Build history of the part. All positions in model axes, mm. Face numbers are marked on the shaded views. Round coordinates to 2 decimals unless told otherwise and drop trailing zeros. Loops run counter-clockwise (first coordinate to the right, second up) from the corner with the lowest first, then second, coordinate; pieces in that order, holes last. Notation, with made-up numbers: (8.5, -15) - (12.5, -15) arc R9 ccw to (12.5, -10) - close; hole circle Ø5 at (61.25, 52.25). An arc over 180 degrees is marked (long way). Put each result on its own line as item: value. Start each with the question number.
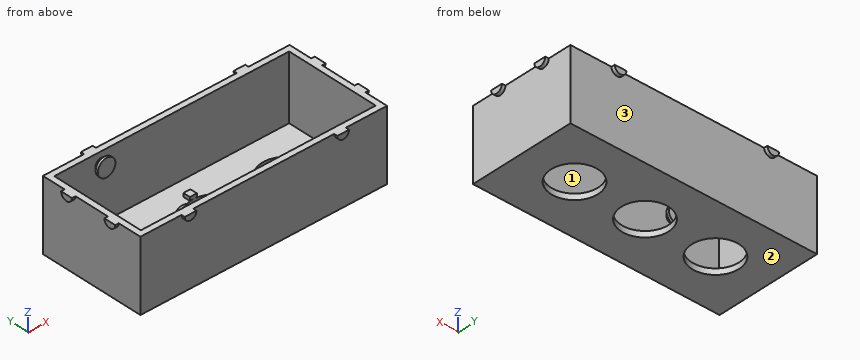
Autodesk Fusion 360 part; units mm, degrees
sketch "Sketch1" plane through (0, 0, 0) normal (0, 0, 1) x (1, 0, 0)
  line L0 (0, 0) -> (210, 0)
  line L1 (210, 0) -> (210, 90)
  line L2 (210, 90) -> (0, 90)
  line L3 (0, 90) -> (0, 0)
  line L4 (5, 5) -> (205, 5)
  line L5 (205, 5) -> (205, 85)
  line L6 (205, 85) -> (5, 85)
  line L7 (5, 85) -> (5, 5)
  circle A0 centre (45, 45) radius 20
  circle A1 centre (105, 45) radius 20
  circle A2 centre (165, 45) radius 20
  dimension "d1" = 210
  dimension "d2" = 90
  dimension "d3" = 200
  dimension "d4" = 80
  dimension "d5" = 5
  dimension "d6" = 5
  dimension "d7" = 40
  dimension "d8" = 40
  dimension "d9" = 40
  dimension "d10" = 105
  dimension "d11" = 45
  dimension "d12" = 45
  dimension "d13" = 45
  dimension "d14" = 60
  dimension "d15" = 60
extrude "Extrude1" add sketch "Sketch1" along normal blind 5 contours L4 L5 L6 L7
extrude "Extrude2" add sketch "Sketch1" along normal blind 60 contours L0 L1 L2 L3
sketch "Sketch2" plane through (210, 0, 0) normal (1, 0, 0) x (0, 1, 0)
  line L0 (0, 0) -> (90, 0)
  line L1 (90, 0) -> (90, 60)
  line L2 (90, 60) -> (0, 60)
  line L3 (0, 60) -> (0, 0)
  circle A0 centre (25, 60) radius 5
  circle A1 centre (65, 60) radius 5
  line L4 (20, 60) -> (30, 60)
  line L5 (60, 60) -> (70, 60)
  dimension "d20" = 10
  dimension "d21" = 10
  dimension "d22" = 25
  dimension "d23" = 25
extrude "Extrude3" add sketch "Sketch2" along normal blind 3 contours L2 A0 L4 | L2 A1 L5 picked at (25.8333, 56.3489) picked at (63.59, 57.0721)
sketch "Sketch3" plane through (0, 0, 0) normal (0, -1, 0) x (1, 0, 0)
  line L0 (0, 0) -> (210, 0)
  line L1 (210, 0) -> (210, 60)
  line L2 (210, 60) -> (0, 60)
  line L3 (0, 60) -> (0, 0)
  circle A0 centre (40, 60) radius 5
  circle A1 centre (170, 60) radius 5
  line L4 (35, 60) -> (45, 60)
  line L5 (165, 60) -> (175, 60)
  dimension "d26" = 10
  dimension "d27" = 10
  dimension "d28" = 40
  dimension "d29" = 40
extrude "Extrude4" add sketch "Sketch3" along normal blind 3 contours L2 A0 L4 | L2 A1 L5 picked at (38.8698, 57.4825) picked at (169.3911, 57.9517)
ref_plane "WorkPlane1" through (105, 45, 30) normal (0, -1, 0) x (1, 0, 0)
ref_plane "WorkPlane2" through (105, 0, 0) normal (1, 0, 0) x (0, 1, 0)
mirror "Mirror1" about plane through (105, 45, 30) normal (0, -1, 0) of bodies 1 merged
mirror "Mirror2" about plane through (105, 0, 0) normal (1, 0, 0) of bodies 1 merged
sketch "Sketch4" plane through (0, 85, 0) normal (0, -1, 0) x (1, 0, 0)
  line L0 (5, 5) -> (205, 5)
  line L1 (205, 5) -> (205, 60)
  line L2 (205, 60) -> (5, 60)
  line L3 (5, 60) -> (5, 5)
  circle A0 centre (45, 50) radius 5
  line L4 (0, 0) -> (0, 60)
  dimension "d38" = 45
  dimension "d39" = 10
extrude "Extrude5" add sketch "Sketch4" along normal blind 5 contours A0
sketch "Sketch5" plane through (0, 80, 0) normal (0, -1, 0) x (1, 0, 0)
  circle A0 centre (45, 50) radius 5
  circle A1 centre (45, 50) radius 7.5
  dimension "d42" = 15
extrude "Extrude6" add sketch "Sketch5" against normal blind 2
mirror "Mirror3" about plane through (105, 45, 30) normal (0, -1, 0) of bodies 1 merged
sketch "Sketch6" plane through (0, 0, 5) normal (0, 0, 1) x (-1, 0, 0)
  arc A0 (-65, -45) -> (-25, -45) centre (-45, -45) ccw
  arc A1 (-25, -45) -> (-65, -45) centre (-45, -45) ccw
  arc A2 (-125, -45) -> (-85, -45) centre (-105, -45) ccw
  arc A3 (-85, -45) -> (-125, -45) centre (-105, -45) ccw
  arc A4 (-185, -45) -> (-145, -45) centre (-165, -45) ccw
  arc A5 (-145, -45) -> (-185, -45) centre (-165, -45) ccw
  line L0 (-5, -85) -> (-5, -5)
  line L1 (-5, -5) -> (-205, -5)
  line L2 (-205, -5) -> (-205, -85)
  line L3 (-205, -85) -> (-5, -85)
  line L4 (-102, -71) -> (-108, -71)
  line L5 (-108, -71) -> (-108, -65)
  line L6 (-108, -65) -> (-102, -65)
  line L7 (-102, -65) -> (-102, -71)
  line L8 (-102, -25) -> (-108, -25)
  line L9 (-108, -25) -> (-108, -19)
  line L10 (-108, -19) -> (-102, -19)
  line L11 (-102, -19) -> (-102, -25)
  circle A6 centre (-105, -45) radius 20
  line L12 (-210, 0) -> (-210, -90)
  line L13 (-102, -71) -> (-108, -71)
  line L14 (-108, -71) -> (-108, -73)
  line L15 (-108, -73) -> (-102, -73)
  line L16 (-102, -73) -> (-102, -71)
  line L17 (-108, -69) -> (-110, -69)
  line L18 (-110, -69) -> (-110, -67)
  line L19 (-110, -67) -> (-108, -67)
  line L20 (-108, -67) -> (-108, -69)
  line L21 (-102, -69) -> (-100, -69)
  line L22 (-100, -69) -> (-100, -67)
  line L23 (-100, -67) -> (-102, -67)
  line L24 (-102, -67) -> (-102, -69)
  line L25 (-108, -19) -> (-102, -19)
  line L26 (-102, -19) -> (-102, -17)
  line L27 (-102, -17) -> (-108, -17)
  line L28 (-108, -17) -> (-108, -19)
  line L29 (-108, -23) -> (-110, -23)
  line L30 (-110, -23) -> (-110, -21)
  line L31 (-110, -21) -> (-108, -21)
  line L32 (-108, -21) -> (-108, -23)
  line L33 (-102, -23) -> (-100, -23)
  line L34 (-100, -23) -> (-100, -21)
  line L35 (-100, -21) -> (-102, -21)
  line L36 (-102, -21) -> (-102, -23)
  dimension "d47" = 6
  dimension "d48" = 6
  dimension "d49" = 6
  dimension "d50" = 6
  dimension "d51" = 102
  dimension "d52" = 2
  dimension "d53" = 2
  dimension "d54" = 2
  dimension "d55" = 2
  dimension "d56" = 2
  dimension "d57" = 2
  dimension "d58" = 2
  dimension "d63" = 6
  dimension "d64" = 2
  dimension "d65" = 2
  dimension "d66" = 2
  dimension "d67" = 2
  dimension "d68" = 2
  dimension "d69" = 2
  dimension "d70" = 2
extrude "Extrude7" add sketch "Sketch6" along normal blind 3 contours L4 L5 L6 L7 L13 L20 L24
extrude "Extrude8" add sketch "Sketch6" along normal blind 2 contours L11 L33 L34 L35 L36 | L9 L29 L30 L31 L32 | L10 L25 L26 L27 L28
1) Slice it at B-B, the plane z = 17. Write the cut outline in (x, y), and give its area (3 significant figures).
2) Slice it at A-A, the plane y = 45. Write the cut outline in (x, z), and give its area (3 significant figures).
3) Pull direction Y, two halves, no side cores. Call the marked faces 1, 2 and 3: pulls with the +Y half, pulls with the -Y half, needs draft (parallel to the pull), parting line crosses it, or undercut.
4) Drop flat-ended pins along their axis: pin 1 Ø5 at (x, z) = (174, 24.5) entering from -Y; pin 2 Ø8 at (y, z) = (13.5, 13) entering from -X; pin 3 Ø0.9 at (y, z) = (66.5, 7) entering from +X. Give the stop position or say it passes through.
5) Drill centre lines: line 1 (X direction, y = 45, z = 3.1); line 2 (Y direction, x = 46.5, z = 18); line 3 (Y direction, x = 165, z = 1.85). Where is each one in solid material? Low to high. Write a range as [from, to].
6) Slice it at D-D, the plane x = 21. Write the cut outline in (y, z), and give its area (3 significant figures).
7) Slice it at C-C, the plane x = 97. Write the cut outline in (y, z), and give its area (3 significant figures).
Taken from the geometry:
1. outline: (0, 0) - (210, 0) - (210, 90) - (0, 90) - close; hole (5, 5) - (205, 5) - (205, 85) - (5, 85) - close
1. area: 2,900 mm2
2. outline: (0, 0) - (25, 0) - (25, 5) - (5, 5) - (5, 60) - (0, 60) - close; (65, 0) - (85, 0) - (85, 5) - (65, 5) - close; (125, 0) - (145, 0) - (145, 5) - (125, 5) - close; (185, 0) - (210, 0) - (210, 60) - (205, 60) - (205, 5) - (185, 5) - close
2. area: 1,000 mm2
3. face 1: undercut
3. face 2: needs draft
3. face 3: pulls with the +Y half
4. pin 1: stops at y = 0
4. pin 2: stops at x = 0
4. pin 3: stops at x = 210
5. line 1: x = [0, 25], [65, 85], [125, 145], [185, 210]
5. line 2: y = [0, 5], [85, 90]
5. line 3: y = [0, 25], [65, 90]
6. outline: (0, 0) - (90, 0) - (90, 60) - (85, 60) - (85, 5) - (5, 5) - (5, 60) - (0, 60) - close
6. area: 1,000 mm2
7. outline: (0, 0) - (26.67, 0) - (26.67, 5) - (5, 5) - (5, 60) - (0, 60) - close; (63.33, 0) - (90, 0) - (90, 60) - (85, 60) - (85, 5) - (63.33, 5) - close
7. area: 817 mm2
